Can you work these out from the drawing? Everything is in mm from the part's minimum corner. A direction names the side the tool comes from. Coordinates: 2 decimals unless noted, no trailing zeros. Write each loop counter-clockwise with the first axis right and the second up, starting at its lowest first coordinate (ties: lowest second). Pieces come first, ordered by that corner, then holes. Notation, with made-up numbers: (11.5, 2) -> (22.5, 2) arc R16 ccw to (22.5, 27) -> close; hole circle Ø1 at (58.5, 23). An arc over 180 degrees is marked (long way). Use a Markdown table: item, result. Add a question column.
Item 1: On a 3-axis mill with a long thin cutter (end or side, diameter ignored), from which of +Z, -Z, +X, -X, +Y, -Y can I reach the whole of each face in a straight line? I mean the marked faces 1 and 2. Say none if no direction works.
Item 2: Imagine slicing it at C-C, the plane y = 158. Write out the boundary of the cut face in (x, z), and give its area (3 significant figures).
Item 3: If I drill on line 1 along X through (y, z) = (103, 114.5); line 2 along Z through (x, y) = (330, 113.5), over which ranges is the centre line in solid material (lowest first)? Write a range as from..to.
Item 4: Imagine slicing it at A-A, the plane z = 121. Write out the boundary of the cut face in (x, y).
Item 5: Imagine slicing it at D-D, the plane x = 172. Write out the boundary of the cut face in (y, z).
Item 6: Imagine slicing it at B-B, the plane y = 97. Write out the boundary of the cut face in (x, z).
Item 7: If we mould it in two halves opening along X, with no side actions, what happens to the marked faces 3, 4 and 5? For each: pulls with the +X half, pulls with the -X half, needs draft (parallel to the pull), parting line crosses it, or undercut.
Item 8: Will these pins go through, and if not, where does the flat tip stop? pin 1 Ø5 at (x, z) = (168, 136.5) entering from -Y; pin 2 Ø4 at (x, y) = (301, 30) entering from -Z; pin 3 Ø11 at (y, z) = (47, 133) entering from -X.
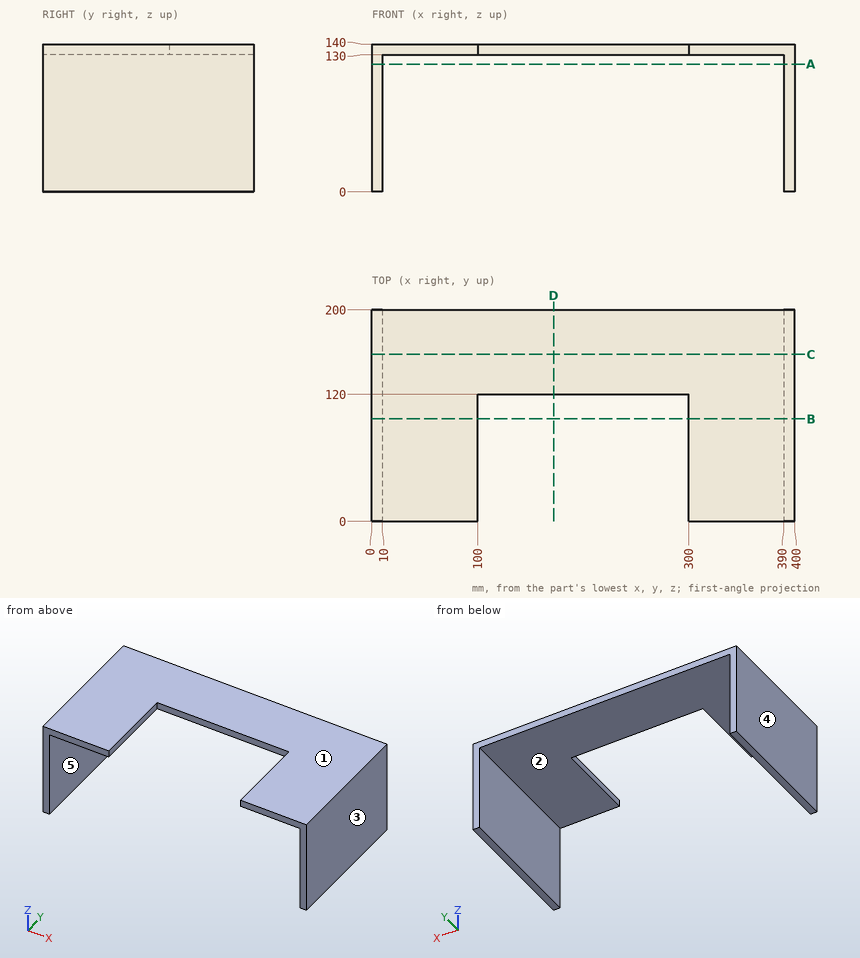
Ans:
| question | item | result |
|---|---|---|
| 1 | face 1 | +Z, +X, -X, +Y, -Y |
| 1 | face 2 | -Z, +Y, -Y |
| 2 | outline | (0, 0) -> (10, 0) -> (10, 130) -> (390, 130) -> (390, 0) -> (400, 0) -> (400, 140) -> (0, 140) -> close |
| 2 | area | 6,600 mm^2 |
| 3 | line 1 | x = 0..10, 390..400 |
| 3 | line 2 | z = 130..140 |
| 4 | outline | (0, 0) -> (10, 0) -> (10, 200) -> (0, 200) -> close; (390, 0) -> (400, 0) -> (400, 200) -> (390, 200) -> close |
| 5 | outline | (120, 130) -> (200, 130) -> (200, 140) -> (120, 140) -> close |
| 6 | outline | (0, 0) -> (10, 0) -> (10, 130) -> (100, 130) -> (100, 140) -> (0, 140) -> close; (300, 130) -> (390, 130) -> (390, 0) -> (400, 0) -> (400, 140) -> (300, 140) -> close |
| 7 | face 3 | pulls with the +X half |
| 7 | face 4 | pulls with the -X half |
| 7 | face 5 | undercut |
| 8 | pin 1 | stops at y = 120 |
| 8 | pin 2 | stops at z = 130 |
| 8 | pin 3 | stops at x = 0 |
